For this review, take the finished solid that the model builds, in its own axes (mm). A direction names the side the tool comes from. Round coordinates to 2 decimals unless told otherwise and drop trailing zeros. Loops run counter-clockwise (first coordinate to the right, second up) from the corner with the lowest first, then second, coordinate; pieces in that order, holes last. Notation, with made-up numbers: (-14.5, 37) -> (21.5, 37) arc R35 ccw to (21.5, 70) -> close; hole circle Ø1 at (-5.75, -4.5). An arc over 180 degrees is marked (long way). Write each question's results on one line, items separated by ' | '.
```python
from build123d import *

# Parameters (mm, degrees)
F0_W     = 27.0002
F0_H     = 58.7502
F1_DEPTH = 6.858
F2_W     = 11.43
F2_H     = 22.86
F3_DEPTH = 69.85
F4_W     = 14.859
F4_H     = 14.859
F5_DEPTH = 76.2


with BuildPart() as f1:
    # F0 (on Top) → F1 (new body)
    with BuildSketch(Plane.XY):
        with Locations((-21.517536, -29.3751)):
            Rectangle(F0_W, F0_H)
    extrude(amount=F1_DEPTH)

    # F2 (on Top) → F3 (join)
    with BuildSketch(Plane.XY):
        with Locations((-27.232536, -11.43)):
            Rectangle(F2_W, F2_H)
        with Locations((-15.802536, -11.43)):
            Rectangle(F2_W, F2_H)
    extrude(amount=F3_DEPTH)

    # F4 (on face) → F5 (cut)
    with BuildSketch(Plane.XY.offset(69.85)):
        with Locations((-21.530236, -11.4427)):
            Rectangle(F4_W, F4_H)
    extrude(amount=-F5_DEPTH, mode=Mode.SUBTRACT)


solid = f1.part
```
1. Consider section D-D (x = -12.5). State the section outline as (y, z) points, plus the area to 3 significant figures.
Values found:
outline: (-58.75, 0) -> (0, 0) -> (0, 69.85) -> (-22.86, 69.85) -> (-22.86, 6.86) -> (-58.75, 6.86) -> close | area: 1,840 mm2
2. Draft analysis for pull direction Y (two halves, no side actions). For faces 1 (the face through (-14.101, -12, 35)), 2 (the face through (-22, -4.013, 35)), 3 (the face through (-8.017, -30, 3)), 4 (the face through (-22, -58.75, 3)), state which applies: released by +Y, released by -Y, zero draft, split by the parting line, or undercut.
Values found:
face 1: undercut | face 2: undercut | face 3: zero draft | face 4: released by -Y
3. For pin 1 (25 mm diameter, centred on y = -8, z = 29, fed in from -X); pin 2 (4.5 mm diameter, centred on y = -12, z = 42.5, fed in from +X); pin 3 (3 mm diameter, centred on x = -24, z = 26.5, fed in from -Y), all flat-tipped, find the tip position at first contact; note any pin that passes through.
Values found:
pin 1: stops at x = -32.95 | pin 2: stops at x = -10.09 | pin 3: stops at y = -22.86
4. Tool access review of faces 5 (the face through (-32.948, -12, 38)), 6 (the face through (-22, -22.86, 38)), 7 (the face through (-10.088, -12, 38)), 8 (the face through (-22, -18.872, 35)): name each direction out of +Z, -Z, +X, -X, +Y, -Y from which nothing blocks a thin tool from reaching the whole face with its end or side.
Values found:
face 5: +Z, -X, +Y, -Y | face 6: +Z, +X, -X, -Y | face 7: +Z, +X, +Y, -Y | face 8: +Z, -Z
5. Consider section A-A (z = 40.5). State the section outline as (x, y) points, plus the area to 3 significant figures.
Values found:
outline: (-32.95, -22.86) -> (-10.09, -22.86) -> (-10.09, 0) -> (-32.95, 0) -> close; hole (-28.96, -18.87) -> (-14.1, -18.87) -> (-14.1, -4.01) -> (-28.96, -4.01) -> close | area: 302 mm2
6. Consider section C-C (y = -13.5). State the section outline as (x, z) points, plus the area to 3 significant figures.
Values found:
outline: (-35.02, 0) -> (-28.96, 0) -> (-28.96, 69.85) -> (-32.95, 69.85) -> (-32.95, 6.86) -> (-35.02, 6.86) -> close; (-14.1, 0) -> (-8.02, 0) -> (-8.02, 6.86) -> (-10.09, 6.86) -> (-10.09, 69.85) -> (-14.1, 69.85) -> close | area: 587 mm2
7. To check wall thickness, follow probe 1 along X at (y, z) = (-11.5, 46.5); probe 2 along Y at (x, z) = (-21.25, 49.5); probe 3 along Y at (x, z) = (-13, 61). State the ranges of each line that lie inside material, in increasing order.
Values found:
probe 1: x = -32.95 to -28.96, -14.1 to -10.09 | probe 2: y = -22.86 to -18.87, -4.01 to 0 | probe 3: y = -22.86 to 0
8. Consider section B-B (x = -24.25). State the section outline as (y, z) points.
Values found:
outline: (-58.75, 0) -> (-18.87, 0) -> (-18.87, 69.85) -> (-22.86, 69.85) -> (-22.86, 6.86) -> (-58.75, 6.86) -> close; (-4.01, 0) -> (0, 0) -> (0, 69.85) -> (-4.01, 69.85) -> close
